```python
from build123d import *


with BuildPart() as f2:
    # F2: sweep along a path in F1
    with BuildLine(Plane.YZ) as f2_path:
        Line((0, 0), (289.022509, 0))
        ThreePointArc((289.022509, 0), (305.092199, 5.848889), (313.642703, 20.658796))
        Line((313.642703, 20.658796), (327.516535, 99.341204))
        ThreePointArc((327.516535, 99.341204), (336.067038, 114.151111), (352.136728, 120))
        Line((352.136728, 120), (521.159238, 120))
    # F0 (on Front) → F2 (sweep)
    with BuildSketch(Plane.XZ):
        Polygon((0.012307, -5.773503), (5.006153, -2.876093), (4.993847, 2.897409), (-0.012307, 5.773503), (-5.006153, 2.876093), (-4.993847, -2.897409), align=None)
    sweep(path=f2_path.line)


solid = f2.part
```
Verification items for the finished model (mm, model axes). Give positions to 0.01 mm unless a question says otherwise; leave off trailing zeros. Order: outer loops, then holes, each group sorted by start corner. A loop starts at its lowest first (then second) coordinate and runs counter-clockwise, first axis right, second up. Notation, with made-up numbers: (68, -23.75) -> (115, -23.75) arc R25 cw to (115, -0.75) -> close; hole circle Ø1 at (55.5, -12). An arc over 180 degrees is marked (long way). One line per item, written item: value.
(1) Sectioned sample at C-C on z = 59.5. Record the cut outline in (x, y).
Final values:
outline: (-5.01, 317.57) -> (-0.01, 314.63) -> (4.99, 317.55) -> (5.01, 323.41) -> (0.01, 326.35) -> (-4.99, 323.43) -> close
(2) Sectioned sample at B-B on y = 234. Record the cut outline in (x, z).
Final values:
outline: (-5.01, 2.88) -> (-4.99, -2.9) -> (0.01, -5.77) -> (5.01, -2.88) -> (4.99, 2.9) -> (-0.01, 5.77) -> close
(3) Scan lines: line 1 along Z through (x, y) = (0, 213.5); line 2 along Z through (x, y) = (1.5, 33); line 3 along Y through (x, z) = (-2, 30.5). Record each from-to range of solid material in increasing order. Write a range as [from, to].
Final values:
line 1: [-5.77, 5.77]
line 2: [-4.91, 4.9]
line 3: [310.69, 320.07]
(4) Gauge pin test, flat ends, axial feed: pin 1 (1.5 mm diameter, centred on x = 2.5, y = 91, fed in from -Z); pin 2 (6 mm diameter, centred on x = -1, y = 158, fed in from +Z); pin 3 (1 mm diameter, centred on x = 3, z = 21, fed in from -Y). Record the tip position at first contact, or that the pin passes through.
Final values:
pin 1: z = -4.77
pin 2: z = 5.77
pin 3: y = 309.28
(5) Sectioned sample at A-A on x = -3.25. Record the cut outline in (y, z) (1 decimal).
Final values:
outline: (0, -3.9) -> (289, -3.9) arc R28.9 ccw to (317.5, 20) -> (331.4, 98.7) arc R21.1 cw to (352.1, 116.1) -> (521.2, 116.1) -> (521.2, 123.9) -> (352.1, 123.9) arc R28.9 ccw to (323.7, 100) -> (309.8, 21.3) arc R21.1 cw to (289, 3.9) -> (0, 3.9) -> close
